Part model, mm, in its own coordinate system. Face numbers are marked on the shaded views. A direction names the side the tool comes from. Coordinates: 2 decimals unless noted, no trailing zeros. Loops run counter-clockwise (first coordinate to the right, second up) from the corner with the lowest first, then second, coordinate; pieces in that order, holes last.
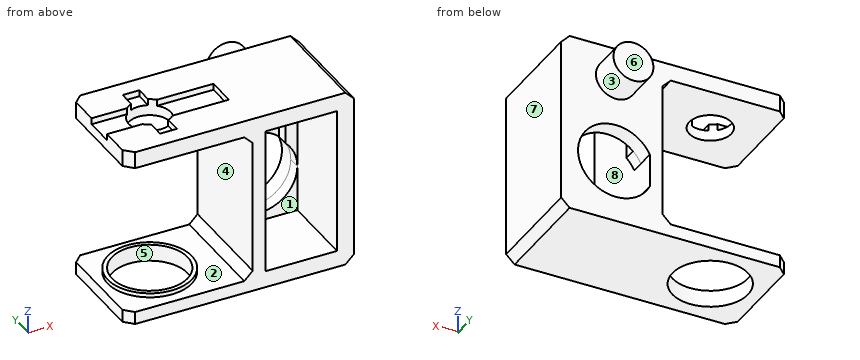
Autodesk Inventor part; units mm, degrees
ref_plane "YZ Plane" through (0, 0, 0) normal (1, 0, 0) x (0, 1, 0)
ref_plane "XZ Plane" through (0, 0, 0) normal (0, 1, 0) x (-1, 0, 0)
ref_plane "XY Plane" through (0, 0, 0) normal (0, 0, 1) x (1, 0, 0)
sketch "Boceto1" plane through (0, 0, 0) normal (0, 1, 0) x (-1, 0, 0)
  line L0 (0, 0) -> (4, 0)
  line L1 (4, 0) -> (4, 43)
  line L2 (4, 43) -> (0, 43)
  line L3 (0, 43) -> (0, 0)
  line L4 (4, 43) -> (54, 43)
  line L5 (54, 43) -> (54, 39)
  line L6 (54, 39) -> (4, 39)
  line L7 (4, 39) -> (4, 43)
  line L8 (4, 0) -> (54, 0)
  line L9 (54, 0) -> (54, 4)
  line L10 (54, 4) -> (4, 4)
  line L11 (4, 4) -> (4, 0)
  dimension "d4" = 43
  dimension "d5" = 50
  dimension "d6" = 4
  dimension "d7" = 50
  dimension "d8" = 4
  dimension "d54" = 4
extrude "Extrusión1" add sketch "Boceto1" along normal blind 25
sketch "Boceto3" plane through (-54, 0, 4) normal (0, 0, 1) x (1, 0, 0)
  line L0 (0, 0) -> (0, 25)
  circle A0 centre (12, 12.5) radius 9
  point P0 (54, 0)
  point P1 (0, 12.5)
  dimension "d19" = 18
  dimension "d20" = 12
extrude "Extrusión2" cut sketch "Boceto3" against normal blind 8 and the other way blind 2
sketch "Boceto8" plane through (-54, 0, 43) normal (0, 0, 1) x (1, 0, 0)
  circle A0 centre (12, 12.5) radius 5
  line L0 (0, 0) -> (0, 25)
  line L1 (0, 9) -> (0, 16)
  point P0 (0, 12.5)
  dimension "d40" = 10
  dimension "d42" = 12
extrude "Extrusión7" cut sketch "Boceto8" against normal blind 5
sketch "Boceto9" plane through (-54, 0, 43) normal (0, 0, 1) x (1, 0, 0)
  circle A0 centre (12, 12.5) radius 5
  line L0 (0, 16) -> (29, 16)
  line L1 (29, 16) -> (29, 9)
  line L2 (29, 9) -> (0, 9)
  line L3 (0, 9) -> (0, 16)
  dimension "d44" = 17
  dimension "d45" = 7
sketch "Boceto10" plane through (-54, 0, 43) normal (0, 0, 1) x (1, 0, 0)
  circle A0 centre (12, 12.5) radius 5
  line L0 (0, 0) -> (0, 25)
  line L1 (10, 21) -> (14, 21)
  line L2 (14, 21) -> (14, 4)
  line L3 (14, 4) -> (10, 4)
  line L4 (10, 4) -> (10, 21)
  point P0 (10, 12.5)
  point P1 (0, 12.5)
  point P2 (12, 21)
  dimension "d48" = 4
  dimension "d49" = 17
extrude "Extrusión8" cut sketch "Boceto10" against normal blind 1.5 contours L2 A0 L4 | A0 L4 L1 L2 | L2 L3 L4 A0
extrude "Extrusión9" cut sketch "Boceto9" against normal blind 1.5 contours A0 L2 L0 | A0 L0 L1 L2 | A0 L2 L3 L0
chamfer "Chaflán1" distance 2 angle 45 1 edges at (0, 12.5, 0)
chamfer "Chaflán2" distance 2 angle 45 1 edges at (0, 12.5, 43)
sketch "Boceto13" plane through (-54, 0, 4) normal (0, 0, 1) x (1, 0, 0)
  line L0 (0, 25) -> (50, 25)
  line L1 (29.9369, 25) -> (49.9369, 25)
  line L2 (49.9369, 25) -> (49.9369, 0)
  line L3 (49.9369, 0) -> (29.9369, 0)
  line L4 (29.9369, 0) -> (29.9369, 25)
  point P0 (54, 0)
  dimension "d80" = 20
  dimension "d81" = 25
extrude "Extrusión12" add sketch "Boceto13" along normal blind 5
sketch "Boceto14" plane through (-54, 0, 9) normal (0, 0, 1) x (1, 0, 0)
  line L0 (49.9369, 25) -> (32.9369, 25)
  line L1 (32.9369, 25) -> (32.9369, -5)
  line L2 (32.9369, -5) -> (49.9369, -5)
  line L3 (49.9369, -5) -> (49.9369, 25)
  dimension "d84" = 17
  dimension "d85" = 30
extrude "Extrusión13" cut sketch "Boceto14" against normal blind 5
sketch "Boceto15" plane through (-4, 0, 4) normal (0, 0, 1) x (1, 0, 0)
  line L0 (0, 25) -> (0, 0)
  line L1 (-17.0631, 25) -> (0, 25)
  line L2 (0, 25) -> (0, 21)
  line L3 (0, 21) -> (-17.0631, 21)
  line L4 (-17.0631, 21) -> (-17.0631, 25)
  point P0 (4, 0)
extrude "Extrusión14" add sketch "Boceto15" along normal up to next
sketch "Boceto16" plane through (0, 25, 0) normal (0, 1, 0) x (1, 0, 0)
  circle A0 centre (-13, -15) radius 9
  line L0 (-21.0631, -4) -> (-4, -4)
  line L1 (-4, -39) -> (-4, -4)
  point P0 (0, 0)
  dimension "d90" = 11
  dimension "d91" = 18
extrude "Extrusión15" cut sketch "Boceto16" against normal blind 5
sketch "Boceto17" plane through (-4, 0, 39) normal (0, 0, -1) x (-1, 0, 0)
  line L0 (0, 0) -> (50, 0)
  line L1 (17.0631, 25) -> (20.0631, 25)
  line L2 (20.0631, 25) -> (20.0631, 0)
  line L3 (20.0631, 0) -> (17.0631, 0)
  line L4 (17.0631, 0) -> (17.0631, 25)
  point P0 (-4, 0)
  dimension "d94" = 3
extrude "Extrusión16" add sketch "Boceto17" along normal up to next
sketch "Boceto18" plane through (0, 25, 0) normal (0, 1, 0) x (1, 0, 0)
  circle A0 centre (-13, -15) radius 9
  line L0 (-54, -43) -> (-2, -43)
  circle A1 centre (-13, -35.3) radius 4.75
  point P0 (0, 0)
  dimension "d97" = 9.5
  dimension "d98" = 7.7
extrude "Extrusión17" add sketch "Boceto18" along normal blind 8 contours A1
sketch "Boceto20" plane through (-21.0631, 21, 39) normal (0, -1, 0) x (1, 0, 0)
  arc A0 (17.0631, -24) -> (0, -20.0018) centre (8.0631, -24) ccw
  line L0 (0, -20.0018) -> (0, 0)
  line L1 (0, 0) -> (17.0631, 0)
  line L2 (17.0631, 0) -> (17.0631, -24)
  line L3 (17.0631, -24) -> (0, -24)
  line L4 (0, -24) -> (0, 0)
  point P0 (21.0631, -39)
extrude "Extrusión19" add sketch "Boceto20" along normal blind 3 contours A0 L0 L1 L2
sketch "Boceto21" plane through (-21.0631, 18, 39) normal (0, -1, 0) x (1, 0, 0)
  arc A0 (17.0631, -24) -> (0, -20.0018) centre (8.0631, -24) ccw
  line L0 (1.9131, -30.2886) -> (14.2131, -30.2886)
  line L1 (14.2131, -30.2886) -> (14.2131, -6.6886)
  line L2 (14.2131, -6.6886) -> (1.9131, -6.6886)
  line L3 (1.9131, -6.6886) -> (1.9131, -30.2886)
  point P0 (21.0631, -39)
  point P1 (8.0631, -30.2886)
  dimension "d108" = 12.3
  dimension "d109" = 23.6
extrude "Extrusión20" cut sketch "Boceto21" against normal blind 3
sketch "Boceto23" plane through (-54, 0, 4) normal (0, 0, 1) x (1, 0, 0)
  circle A0 centre (12, 12.5) radius 9
  line L0 (29.9369, 0) -> (29.9369, 25)
  line L1 (0, 25) -> (29.9369, 25)
  line L2 (0, 0) -> (0, 25)
  line L3 (0, 0) -> (29.9369, 0)
  circle A1 centre (12, 12.5) radius 10
  point P0 (54, 0)
  dimension "d114" = 20
extrude "Extrusión22" cut sketch "Boceto23" against normal blind 1 contours L3 L2 L1 L0
sketch "Boceto24" plane through (-13, 21, 4) normal (0, -1, 0) x (1, 0, 0)
  arc A0 (0, 0) -> (9, 11) centre (0, 9) ccw
  line L0 (9, 0) -> (-8.0631, 0)
  line L1 (9, 11) -> (9, 0)
  point P0 (13, -4)
sketch "Boceto25" plane through (-21.0631, 21, 4) normal (0, -1, 0) x (1, 0, 0)
  arc A0 (0, 7.0018) -> (17.0631, 11) centre (8.0631, 11) ccw
  line L0 (0, 0) -> (0, 7.0018)
  line L1 (17.0631, 0) -> (0, 0)
  point P0 (8.0631, 0)
  point P1 (21.0631, -4)
sketch "Boceto26" plane through (-21.0631, 21, 4) normal (0, -1, 0) x (1, 0, 0)
  arc A0 (0, 7.0018) -> (17.0631, 11) centre (8.0631, 11) ccw
  line L0 (0, 0) -> (0, 7.0018)
  line L1 (17.0631, 0) -> (0, 0)
  line L2 (17.0631, 11) -> (17.0631, 0)
  point P0 (21.0631, -4)
extrude "Extrusión25" add sketch "Boceto26" along normal blind 3
chamfer "Chaflán5" distance 2 angle 45 2 edges at (-24.0631, 12.5, 3) (-24.0631, 12.5, 39)
chamfer "Chaflán6" distance 2 angle 45 4 edges at (-54, 0, 41) (-54, 25, 41) (-54, 25, 1.5) (-54, 0, 1.5)
properties part number "Pinza"
Q1. Saw through at D-D (y = 6). List the corners of the cut face in (x, z), plus the area to 3 significant figures.
Q2. Saw through at C-C (z = 16.5). List the corners of the cut face in (x, y).
Q3. Tool access for the marked faces 1, 2, 3, 4 and 5: list every direction of +Z, -Z, +X, -X, +Y, -Y with a clear straight run to the whole face (end or side of a thin tool).
Q4. Probe line 1 (X direction, y = 23, z = 15); line 2 (Z direction, x = -51, y = 14); line 3 (Z direction, x = -19, y = 14). List the from-to ranges inside material, lowest first.
Q5. Saw through at A-A (y = 12.5). Count the separate pieces of the cut face and the enclosed holes in it, plus the area to 3 significant figures.
Q6. Saw through at B-B (x = -29.5). List the corners of the cut face in (y, z).
Q7. Mould opens along X. For the marked faces 6, 7 and 8 say: released by +X, released by -X, zero draft, split by the parting line, or undercut.
Q8. Drop flat-ended pins along their axis: P1, Ø0.8, axis at y = 14, z = 42.5, coming from the -X side; P2, Ø4, axis at y = 12.5, z = 34.5, coming from the -X side; P3, Ø1.6, axis at y = 19, z = 42.5, coming from the +X side. Give the stop position or say it passes through.
Checked values:
1. outline: (-54, 0) - (-48.22, 0) - (-48.22, 4) - (-49.6, 4) - (-49.6, 3) - (-54, 3) - close; (-54, 39) - (-26.06, 39) - (-24.06, 37) - (-24.06, 5) - (-26.06, 3) - (-34.4, 3) - (-34.4, 4) - (-35.78, 4) - (-35.78, 0) - (-2, 0) - (0, 2) - (0, 41) - (-2, 43) - (-40, 43) - (-40, 41.5) - (-44, 41.5) - (-44, 43) - (-54, 43) - close; hole (-21.06, 4) - (-4, 4) - (-4, 39) - (-21.06, 39) - close
1. area: 606 mm2
2. outline: (-24.06, 0) - (-21.06, 0) - (-21.06, 25) - (-24.06, 25) - close; (-4.13, 18) - (-4, 18) - (-4, 0) - (0, 0) - (0, 25) - (-4.13, 25) - close
3. face 1: -Y
3. face 2: none
3. face 3: +Y
3. face 4: -X, +Y, -Y
3. face 5: -Z
4. line 1: x = -24.06 to -21.06, -4 to 0
4. line 2: z = 0 to 4, 39 to 41.5
4. line 3: z = 0 to 4, 39 to 43
5. separate pieces: 3
5. enclosed holes: 1
5. area: 527 mm2
6. outline: (0, 0) - (25, 0) - (25, 3) - (0, 3) - close; (0, 39) - (25, 39) - (25, 43) - (16, 43) - (16, 41.5) - (9, 41.5) - (9, 43) - (0, 43) - close
7. face 6: zero draft
7. face 7: released by +X
7. face 8: undercut
8. P1: stops at x = -25
8. P2: stops at x = -24.06
8. P3: stops at x = -0.7
